Geometry: final body of the model. Coordinates: model frame, mm. Coordinates: 2 decimals unless noted, no trailing zeros. Write each loop counter-clockwise with the first axis right and the second up, starting at its lowest first coordinate (ties: lowest second). Pieces come first, ordered by that corner, then holes. Notation, with made-up numbers: (-16, 56) - (-9, 56) arc R28 ccw to (-9, 79) - close; hole circle Ø6 at (83.5, -12.5). An arc over 180 degrees is marked (long way). Put each result on its own line as item: value.
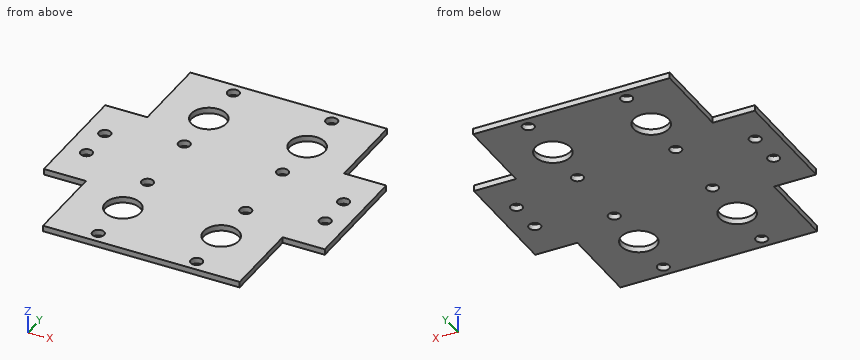
```python
from build123d import *

# Parameters (mm, degrees)
SKETCH1_W           = 240
SKETCH1_H           = 100
BOSS_EXTRUDE1_DEPTH = 5
SKETCH2_W           = 168
SKETCH2_H           = 240
BOSS_EXTRUDE2_DEPTH = 5
SKETCH3_R           = 5
CUT_EXTRUDE1_DEPTH  = 5
SKETCH4_R           = 15
SKETCH4_R_2         = 5
CUT_EXTRUDE2_DEPTH  = 5


with BuildPart() as part:
    # Sketch1 → Boss-Extrude1 (new body)
    with BuildSketch(Plane.XY):
        Rectangle(SKETCH1_W, SKETCH1_H)
    extrude(amount=BOSS_EXTRUDE1_DEPTH)

    # Sketch2 → Boss-Extrude2 (add)
    with BuildSketch(Plane.XY.offset(5)):
        Rectangle(SKETCH2_W, SKETCH2_H)
    extrude(amount=-BOSS_EXTRUDE2_DEPTH)

    # Sketch3 → Cut-Extrude1 (cut)
    with BuildSketch(Plane.XY.offset(5)):
        with Locations((-102, 15)):
            Circle(SKETCH3_R)
        with Locations((102, 15)):
            Circle(SKETCH3_R)
        with Locations((102, -15)):
            Circle(SKETCH3_R)
        with Locations((-102, -15)):
            Circle(SKETCH3_R)
    extrude(amount=-CUT_EXTRUDE1_DEPTH, mode=Mode.SUBTRACT)

    # Sketch4 → Cut-Extrude2 (cut)
    with BuildSketch(Plane.XY.offset(5)):
        with Locations((-42, -70)):
            Circle(SKETCH4_R)
        with Locations((42, -70)):
            Circle(SKETCH4_R)
        with Locations((-42, -30)):
            Circle(SKETCH4_R_2)
        with Locations((-42, -110)):
            Circle(SKETCH4_R_2)
        with Locations((42, -110)):
            Circle(SKETCH4_R_2)
        with Locations((42, -30)):
            Circle(SKETCH4_R_2)
        with Locations((42, 30)):
            Circle(SKETCH4_R_2)
        with Locations((42, 110)):
            Circle(SKETCH4_R_2)
        with Locations((-42, 110)):
            Circle(SKETCH4_R_2)
        with Locations((-42, 30)):
            Circle(SKETCH4_R_2)
        with Locations((42, 70)):
            Circle(SKETCH4_R)
        with Locations((-42, 70)):
            Circle(SKETCH4_R)
    extrude(amount=-CUT_EXTRUDE2_DEPTH, mode=Mode.SUBTRACT)


solid = part.part
```
1. Pin query (flat end, axial travel): pin 1 Ø3 at (x, z) = (91.5, 2) entering from +Y; pin 2 Ø3 at (y, z) = (52, 4) entering from -X; pin 3 Ø11.5 at (x, y) = (42, -30) entering from -Z; pin 4 Ø1.5 at (y, z) = (-84.5, 2.5) entering from +X. Return the tip coordinate at first contact, or that it passes through.
Answer below:
pin 1: stops at y = 50
pin 2: stops at x = -84
pin 3: stops at z = 0
pin 4: stops at x = 84
2. Section query A-A (x = -42). Return loops of the section in (y, z).
Answer below:
outline: (-120, 0) - (-115, 0) - (-115, 5) - (-120, 5) - close; (-105, 0) - (-85, 0) - (-85, 5) - (-105, 5) - close; (-55, 0) - (-35, 0) - (-35, 5) - (-55, 5) - close; (-25, 0) - (25, 0) - (25, 5) - (-25, 5) - close; (35, 0) - (55, 0) - (55, 5) - (35, 5) - close; (85, 0) - (105, 0) - (105, 5) - (85, 5) - close; (115, 0) - (120, 0) - (120, 5) - (115, 5) - close
3. Section query D-D (x = -102). Return loops of the section in (y, z).
Answer below:
outline: (-50, 0) - (-20, 0) - (-20, 5) - (-50, 5) - close; (-10, 0) - (10, 0) - (10, 5) - (-10, 5) - close; (20, 0) - (50, 0) - (50, 5) - (20, 5) - close
4. Section query C-C (z = 0.95). Count the separate pieces of the cut face and the enclosed holes in it, then the cut area to 4 significant figures.
Answer below:
separate pieces: 1
enclosed holes: 16
area: 43,750 mm²
5. Ray query, probe 1 along Y at (x, z) = (-102, 2.4); probe 2 along X at (y, z) = (-70.5, 1.55); probe 3 along X at (y, z) = (75.5, 2.75). Return the intervals inside material, ascending. Write a range as from..to.
Answer below:
probe 1: y = -50..-20, -10..10, 20..50
probe 2: x = -84..-56.99, -27.01..27.01, 56.99..84
probe 3: x = -84..-55.96, -28.04..28.04, 55.96..84
6. Section query B-B (y = 82). Return loops of the section in (x, z), then the cut area to 3 significant figures.
Answer below:
outline: (-84, 0) - (-51, 0) - (-51, 5) - (-84, 5) - close; (-33, 0) - (33, 0) - (33, 5) - (-33, 5) - close; (51, 0) - (84, 0) - (84, 5) - (51, 5) - close
area: 660 mm²
